from build123d import *

# Parameters (mm, degrees)
SKETCH1_R           = 19
SKETCH1_R_2         = 6
BOSS_EXTRUDE1_DEPTH = 16
SKETCH2_R           = 8.265
SKETCH2_R_2         = 6
BOSS_EXTRUDE2_DEPTH = 4
FILLET1_R           = 1
CUT_EXTRUDE1_REACH  = 57.716
SKETCH3_R           = 3.35


with BuildPart() as part:
    # Sketch1 → Boss-Extrude1 (new body)
    # profile 1 of 3: a face of its own
    with BuildSketch(Plane.XY):
        with BuildLine():
            Line((-35.5, -13), (-35.5, -19))
            Line((-35.5, -19), (-3.6e-08, -19))
            ThreePointArc((-3.6e-08, -19), (-13.435028855, -13.43502883), (-19, 0))
            Line((-19, 0), (-19.9, -13))
            Line((-19.9, -13), (-35.5, -13))
        make_face()
    # profile 2 of 3: a face of its own
    with BuildSketch(Plane.XY):
        Circle(SKETCH1_R)
        Circle(SKETCH1_R_2, mode=Mode.SUBTRACT)
    # profile 3 of 3: a face of its own
    with BuildSketch(Plane.XY):
        with BuildLine():
            ThreePointArc((19, 0), (13.43502883, -13.435028855), (-3.6e-08, -19))
            Line((-3.6e-08, -19), (35.5, -19))
            Line((35.5, -19), (35.5, -13))
            Line((35.5, -13), (19.9, -13))
            Line((19.9, -13), (19, 0))
        make_face()
    extrude(amount=BOSS_EXTRUDE1_DEPTH)

    # Sketch2 → Boss-Extrude2 (add)
    with BuildSketch(Plane.XY.offset(16)):
        Circle(SKETCH2_R)
        Circle(SKETCH2_R_2, mode=Mode.SUBTRACT)
    extrude(amount=BOSS_EXTRUDE2_DEPTH)

    # Fillet1
    fillet1_edges = [part.edges().sort_by_distance(p)[0] for p in [
        (-35.5, -13, 8),
        (-19.9, -13, 8),
        (19.9, -13, 8),
        (35.5, -13, 8),
    ]]
    fillet(fillet1_edges, radius=FILLET1_R)

    # Sketch3 → Cut-Extrude1 (cut, up to next)
    with BuildSketch(Plane.XZ.offset(19), mode=Mode.PRIVATE) as cut_extrude1_sk1:
        with Locations(Location((28, 8, 0), (0, 0, 270))):
            Circle(SKETCH3_R)
    cut_extrude1_tool1 = extrude(cut_extrude1_sk1.sketch, amount=-CUT_EXTRUDE1_REACH, mode=Mode.PRIVATE) & part.part
    # Sketch3 → Cut-Extrude1 (cut, up to next)
    with BuildSketch(Plane.XZ.offset(19), mode=Mode.PRIVATE) as cut_extrude1_sk2:
        with Locations(Location((-28, 8, 0), (0, 0, 90))):
            Circle(SKETCH3_R)
    cut_extrude1_tool2 = extrude(cut_extrude1_sk2.sketch, amount=-CUT_EXTRUDE1_REACH, mode=Mode.PRIVATE) & part.part
    add(cut_extrude1_tool1.solids().sort_by_distance((28, -19, 8))[0], mode=Mode.SUBTRACT)
    add(cut_extrude1_tool2.solids().sort_by_distance((-28, -19, 8))[0], mode=Mode.SUBTRACT)


solid = part.part
Build history of the part. All positions in model axes, mm. A direction names the side the tool comes from. Round coordinates to 2 decimals unless told otherwise and drop trailing zeros. Order: outer loops, then holes, each group sorted by start corner. A loop starts at its lowest first (then second) coordinate and runs counter-clockwise, first axis right, second up. Notation, with made-up numbers: M 4,43.5 L 28,43.5 A19 cw 28,55.5 Z; hole C 80.25,-30.75 d7. An arc over 180 degrees is marked long. Use CSV: the item, a comma, the result in double quotes. Start each with the question number.
(1) Cut at B-B on x = 0. List the corners of the cut face in (y, z) (3 decimals).
(2) Cut at C-C on z = 3. List the corners of the cut face in (x, y).
(3) Flat gauge pins, fed straight in: P1, Ø6, axis at x = -28, z = 8, coming from the +Y side; P2, Ø10.5, axis at x = 28, z = 8, coming from the +Y side; P3, Ø1.5, axis at x = -5.5, z = 14.5, coming from the +Y side; P4, Ø1, axis at x = 12, z = 7.5, coming from the +Y side. Where does each tip first touch, or does it go through?
(4) Mould opens along X. For faces 1 (the face through (-19.41, -5.95, 7.89)), 2 (the face through (31.32, -16.04, 8.44)), 3 (the face through (0, -8, 0)) say: +X half, -X half, draft (parallel to the pull), parting line (faces both ways), or undercut.
(5) Tool access for faces 4 (the face through (-24.5, -13, 7.9)), 5 (the face through (35.5, -17, 8)), 6 (the face through (7.883, 2.483, 17.972)), 7 (the face through (25, -13, 6)): list every direction of +Z, -Z, +X, -X, +Y, -Y with a clear straight run to the whole face (end or side of a thin tool).
(6) Cut at D-D on x = 28. List the corners of the cut face in (y, z), then the cut area to 3 significant figures.
(7) Cut at A-A on z = 8. List the corners of the cut face in (x, y).
(8) Drill centre lines: probe 1 along X at (y, z) = (-14.5, 8); probe 2 along Z at (x, y) = (-14.5, 8); probe 3 along X at (y, z) = (-0.5, 9). Where is each one in solid material? Low to high.
Findings:
1,outline,"M -19,0 L -6,0 L -6,20 L -8.265,20 L -8.265,16 L -19,16 Z; M 6,0 L 19,0 L 19,16 L 8.265,16 L 8.265,20 L 6,20 Z"
2,outline,"M -35.5,-19 L 35.5,-19 L 35.5,-14 A1 ccw 34.5,-13 L 20.83,-13 A1 cw 19.84,-12.07 L 19,0 A19 ccw -19,0 L -19.84,-12.07 A1 cw -20.83,-13 L -34.5,-13 A1 ccw -35.5,-14 Z; hole C 0,0 d12"
3,P1,"passes through"
3,P2,"stops at y = -13"
3,P3,"stops at y = 18.4"
3,P4,"stops at y = 15.12"
4,face 1,"-X half"
4,face 2,"undercut"
4,face 3,"draft"
5,face 4,"+Z, -Z, -X, +Y"
5,face 5,"+Z, -Z, +X, +Y, -Y"
5,face 6,"+Z"
5,face 7,"+Z, -Z, +X, +Y"
6,outline,"M -19,0 L -13,0 L -13,4.65 L -19,4.65 Z; M -19,11.35 L -13,11.35 L -13,16 L -19,16 Z"
6,area,"55.8 mm^2"
7,outline,"M -35.5,-19 L -31.35,-19 L -31.35,-13 L -34.5,-13 A1 ccw -35.5,-14 Z; M -24.65,-19 L 24.65,-19 L 24.65,-13 L 20.83,-13 A1 cw 19.84,-12.07 L 19,0 A19 ccw -19,0 L -19.84,-12.07 A1 cw -20.83,-13 L -24.65,-13 Z; M 31.35,-19 L 35.5,-19 L 35.5,-14 A1 ccw 34.5,-13 L 31.35,-13 Z; hole C 0,0 d12"
8,probe 1,"x = -35.5 to -31.35, -24.65 to 24.65, 31.35 to 35.5"
8,probe 2,"z = 0 to 16"
8,probe 3,"x = -19.03 to -5.98, 5.98 to 19.03"
